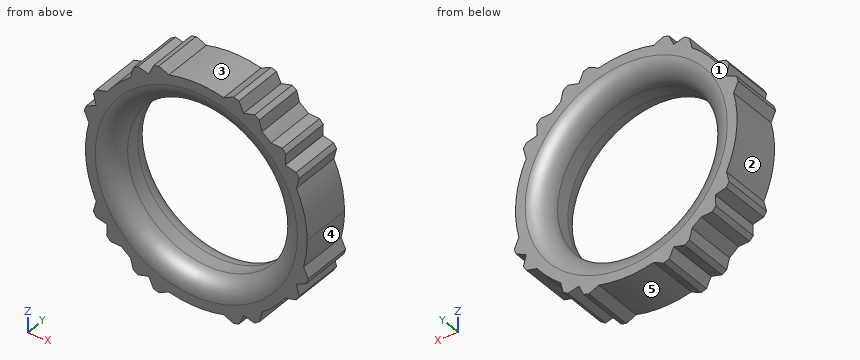
```python
from build123d import *

# Parameters (mm, degrees)
F0_R     = 11.125
F1_DEPTH = 7
F2_R     = 2.54


with BuildPart() as f1:
    # F0 (on Front) → F1 (new body)
    with BuildSketch(Plane.XZ):
        with BuildLine():
            ThreePointArc((14.511314, -3.709508), (14.860825, -1.869371), (14.97794, 0))
            ThreePointArc((14.97794, 0), (14.612658, 3.28769), (13.53463, 6.415019))
            ThreePointArc((13.53463, 6.415019), (12.856111, 7.684991), (12.058783, 8.883942))
            Line((12.058783, 8.883942), (12.034945, 8.889992))
            Line((12.034945, 8.889992), (12.03617, 8.914555))
            ThreePointArc((12.03617, 8.914555), (11.124567, 10.029093), (10.110156, 11.050947))
            ThreePointArc((10.110156, 11.050947), (9.510409, 11.57112), (8.883942, 12.058783))
            ThreePointArc((8.883942, 12.058783), (7.684991, 12.856111), (6.415019, 13.53463))
            ThreePointArc((6.415019, 13.53463), (5.085764, 14.088069), (3.709508, 14.511314))
            ThreePointArc((3.709508, 14.511314), (0, 14.97794), (-3.709508, 14.511314))
            ThreePointArc((-3.709508, 14.511314), (-5.085764, 14.088069), (-6.415019, 13.53463))
            ThreePointArc((-6.415019, 13.53463), (-7.684991, 12.856111), (-8.883942, 12.058783))
            ThreePointArc((-8.883942, 12.058783), (-10.591003, 10.591003), (-12.058783, 8.883942))
            ThreePointArc((-12.058783, 8.883942), (-12.856111, 7.684991), (-13.53463, 6.415019))
            ThreePointArc((-13.53463, 6.415019), (-14.088069, 5.085764), (-14.511314, 3.709508))
            ThreePointArc((-14.511314, 3.709508), (-14.908731, -1.438202), (-13.53463, -6.415019))
            ThreePointArc((-13.53463, -6.415019), (-12.856111, -7.684991), (-12.058783, -8.883942))
            Line((-12.058783, -8.883942), (-12.034945, -8.889992))
            Line((-12.034945, -8.889992), (-12.03617, -8.914555))
            ThreePointArc((-12.03617, -8.914555), (-11.124567, -10.029093), (-10.110156, -11.050947))
            ThreePointArc((-10.110156, -11.050947), (-9.510409, -11.57112), (-8.883942, -12.058783))
            ThreePointArc((-8.883942, -12.058783), (-7.684991, -12.856111), (-6.415019, -13.53463))
            ThreePointArc((-6.415019, -13.53463), (-5.085764, -14.088069), (-3.709508, -14.511314))
            ThreePointArc((-3.709508, -14.511314), (0, -14.97794), (3.709508, -14.511314))
            ThreePointArc((3.709508, -14.511314), (5.085764, -14.088069), (6.415019, -13.53463))
            ThreePointArc((6.415019, -13.53463), (7.684991, -12.856111), (8.883942, -12.058783))
            ThreePointArc((8.883942, -12.058783), (10.591003, -10.591003), (12.058783, -8.883942))
            ThreePointArc((12.058783, -8.883942), (12.856111, -7.684991), (13.53463, -6.415019))
            ThreePointArc((13.53463, -6.415019), (14.088069, -5.085764), (14.511314, -3.709508))
        make_face()
        Circle(F0_R, mode=Mode.SUBTRACT)
        with BuildLine():
            Line((-11.6164, -10.975811), (-10.110156, -11.050947))
            ThreePointArc((-10.110156, -11.050947), (-11.124567, -10.029093), (-12.03617, -8.914555))
            Line((-12.03617, -8.914555), (-12.110081, -10.396236))
            Line((-12.110081, -10.396236), (-11.6164, -10.975811))
        make_face()
        with BuildLine():
            Line((-13.49673, -8.519042), (-12.058783, -8.883942))
            ThreePointArc((-12.058783, -8.883942), (-12.856111, -7.684991), (-13.53463, -6.415019))
            Line((-13.53463, -6.415019), (-13.905579, -7.876804))
            Line((-13.905579, -7.876804), (-13.49673, -8.519042))
        make_face()
        with BuildLine():
            Line((-7.876804, -13.905579), (-6.415019, -13.53463))
            ThreePointArc((-6.415019, -13.53463), (-7.684991, -12.856111), (-8.883942, -12.058783))
            Line((-8.883942, -12.058783), (-8.519042, -13.49673))
            Line((-8.519042, -13.49673), (-7.876804, -13.905579))
        make_face()
        with BuildLine():
            Line((-5.05358, -15.139258), (-3.709508, -14.511314))
            ThreePointArc((-3.709508, -14.511314), (-5.085764, -14.088069), (-6.415019, -13.53463))
            Line((-6.415019, -13.53463), (-5.776666, -14.900984))
            Line((-5.776666, -14.900984), (-5.05358, -15.139258))
        make_face()
        with BuildLine():
            Line((5.776666, -14.900984), (6.415019, -13.53463))
            ThreePointArc((6.415019, -13.53463), (5.085764, -14.088069), (3.709508, -14.511314))
            Line((3.709508, -14.511314), (5.05358, -15.139258))
            Line((5.05358, -15.139258), (5.776666, -14.900984))
        make_face()
        with BuildLine():
            Line((8.519042, -13.49673), (8.883942, -12.058783))
            ThreePointArc((8.883942, -12.058783), (7.684991, -12.856111), (6.415019, -13.53463))
            Line((6.415019, -13.53463), (7.876804, -13.905579))
            Line((7.876804, -13.905579), (8.519042, -13.49673))
        make_face()
        with BuildLine():
            Line((13.905579, -7.876804), (13.53463, -6.415019))
            ThreePointArc((13.53463, -6.415019), (12.856111, -7.684991), (12.058783, -8.883942))
            Line((12.058783, -8.883942), (13.49673, -8.519042))
            Line((13.49673, -8.519042), (13.905579, -7.876804))
        make_face()
        with BuildLine():
            Line((15.139258, -5.05358), (14.511314, -3.709508))
            ThreePointArc((14.511314, -3.709508), (14.088069, -5.085764), (13.53463, -6.415019))
            Line((13.53463, -6.415019), (14.900984, -5.776666))
            Line((14.900984, -5.776666), (15.139258, -5.05358))
        make_face()
        with BuildLine():
            ThreePointArc((-14.511314, 3.709508), (-14.088069, 5.085764), (-13.53463, 6.415019))
            Line((-13.53463, 6.415019), (-14.900984, 5.776666))
            Line((-14.900984, 5.776666), (-15.139258, 5.05358))
            Line((-15.139258, 5.05358), (-14.511314, 3.709508))
        make_face()
        with BuildLine():
            ThreePointArc((-13.53463, 6.415019), (-12.856111, 7.684991), (-12.058783, 8.883942))
            Line((-12.058783, 8.883942), (-13.49673, 8.519042))
            Line((-13.49673, 8.519042), (-13.905579, 7.876804))
            Line((-13.905579, 7.876804), (-13.53463, 6.415019))
        make_face()
        with BuildLine():
            ThreePointArc((12.058783, 8.883942), (12.856111, 7.684991), (13.53463, 6.415019))
            Line((13.53463, 6.415019), (13.905579, 7.876804))
            Line((13.905579, 7.876804), (13.49673, 8.519042))
            Line((13.49673, 8.519042), (12.058783, 8.883942))
        make_face()
        with BuildLine():
            ThreePointArc((10.110156, 11.050947), (11.124567, 10.029093), (12.03617, 8.914555))
            Line((12.03617, 8.914555), (12.110081, 10.396236))
            Line((12.110081, 10.396236), (11.6164, 10.975811))
            Line((11.6164, 10.975811), (10.110156, 11.050947))
        make_face()
        with BuildLine():
            ThreePointArc((6.415019, 13.53463), (7.684991, 12.856111), (8.883942, 12.058783))
            Line((8.883942, 12.058783), (8.519042, 13.49673))
            Line((8.519042, 13.49673), (7.876804, 13.905579))
            Line((7.876804, 13.905579), (6.415019, 13.53463))
        make_face()
        with BuildLine():
            ThreePointArc((3.709508, 14.511314), (5.085764, 14.088069), (6.415019, 13.53463))
            Line((6.415019, 13.53463), (5.776666, 14.900984))
            Line((5.776666, 14.900984), (5.05358, 15.139258))
            Line((5.05358, 15.139258), (3.709508, 14.511314))
        make_face()
        with BuildLine():
            ThreePointArc((-6.415019, 13.53463), (-5.085764, 14.088069), (-3.709508, 14.511314))
            Line((-3.709508, 14.511314), (-5.05358, 15.139258))
            Line((-5.05358, 15.139258), (-5.776666, 14.900984))
            Line((-5.776666, 14.900984), (-6.415019, 13.53463))
        make_face()
        with BuildLine():
            ThreePointArc((-8.883942, 12.058783), (-7.684991, 12.856111), (-6.415019, 13.53463))
            Line((-6.415019, 13.53463), (-7.876804, 13.905579))
            Line((-7.876804, 13.905579), (-8.519042, 13.49673))
            Line((-8.519042, 13.49673), (-8.883942, 12.058783))
        make_face()
    extrude(amount=F1_DEPTH)

    # F2
    f2_edges = [f1.edges().sort_by_distance(p)[0] for p in [
        (-11.125, -7, 0),
        (-11.125, 0, 0),
    ]]
    fillet(f2_edges, radius=F2_R)


solid = f1.part
```
Geometry: final body of the model. Coordinates: model frame, mm. Face numbers are marked on the shaded views. A direction names the side the tool comes from. Round coordinates to 2 decimals unless told otherwise and drop trailing zeros. Order: outer loops, then holes, each group sorted by start corner. A loop starts at its lowest first (then second) coordinate and runs counter-clockwise, first axis right, second up. Notation, with made-up numbers: M 58.25,77.25 L 105.25,77.25 A27 cw 105.25,94.25 Z; hole C -34.75,50.5 d10. An arc over 180 degrees is marked long. One line per item, written item: value.
(1) Reachability of the marked faces 4 and 5 from +Z, -Z, +X, -X, +Y, -Y: full face, straight path, thin tool, end or side. Return the list, or none.
Result sheet:
face 4: +X, +Y, -Y
face 5: -Z, +Y, -Y
(2) Cut plane A-A (x = 0). Return the cut outline in (y, z) (3 decimals), and give its area (3 significant figures).
Result sheet:
outline: M -7,-14.978 L 0,-14.978 L 0,-13.665 A2.54 ccw -2.54,-11.125 L -4.46,-11.125 A2.54 ccw -7,-13.665 Z; M -7,13.665 A2.54 ccw -4.46,11.125 L -2.54,11.125 A2.54 ccw 0,13.665 L 0,14.978 L -7,14.978 Z
area: 48.4 mm2
(3) Line query: probe 1 along Z at (x, y) = (0, -3.3) (3 decimals); probe 2 along X at (y, z) = (-5, -7); probe 3 along Z at (x, y) = (-3, -6.25). Output: solid intervals per line, ascending. Write a range as [from, to].
Result sheet:
probe 1: [-14.978, -11.125], [11.125, 14.978]
probe 2: [-13.68, -8.72], [8.72, 13.68]
probe 3: [-14.67, -11.48], [11.48, 14.67]
(4) Pin query (flat end, axial travel): P1, Ø1.5, axis at y = -4, z = 8, coming from the -X side; P2, Ø1.5, axis at x = -4, y = -4, coming from the -Z side. Return the tip coordinate at first contact, or that it passes through.
Result sheet:
P1: x = -13.91
P2: z = -15
(5) Pull-direction query (Z, two-part tool) for the marked faces 1, 2 and 3; classes: pulls with the +Z half, pulls with the -Z half, needs draft (parallel to the pull), parting line crosses it, or undercut.
Result sheet:
face 1: needs draft
face 2: undercut
face 3: pulls with the +Z half
